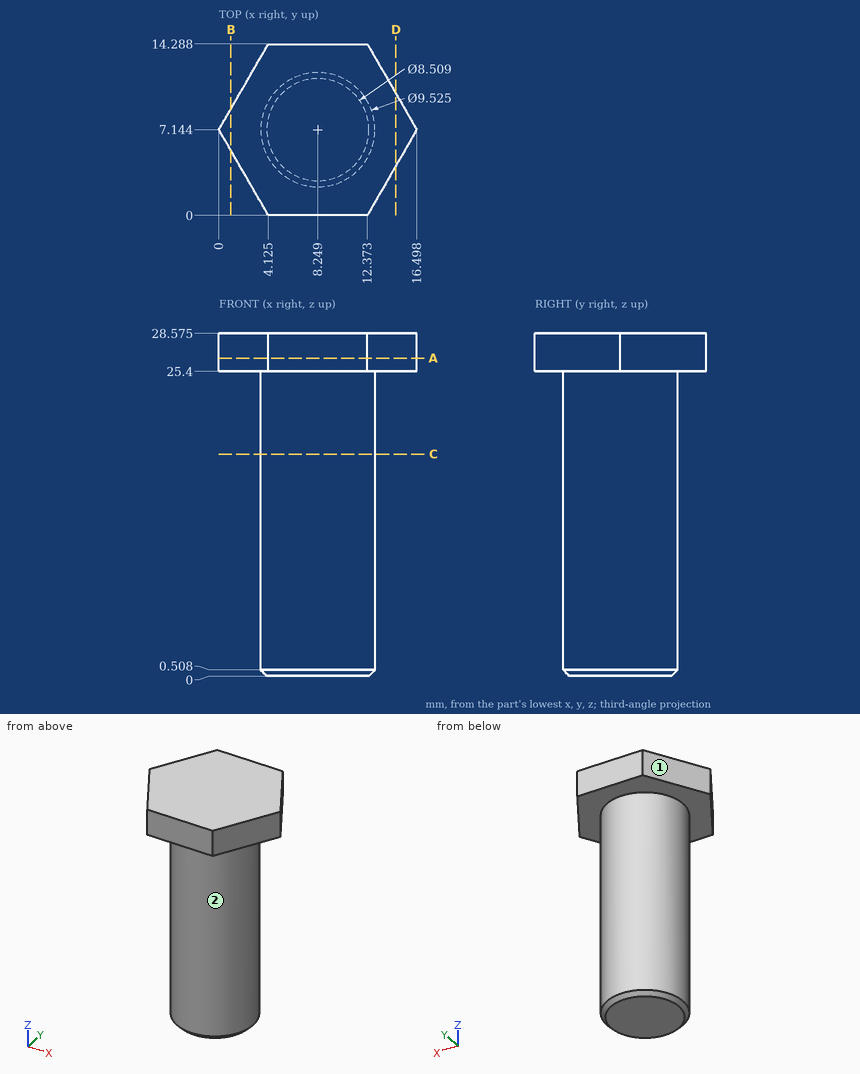
Part print with two shaded views. Sizes in mm from the minimum x, y, z corner. A direction names the side the tool comes from. Round coordinates to 2 decimals unless told otherwise and drop trailing zeros. Write each loop counter-clockwise with the first axis right and the second up, starting at its lowest first coordinate (ties: lowest second). Pieces come first, ordered by that corner, then holes. Notation, with made-up numbers: M 0,27.5 L 18,27.5 A26 cw 18,56.5 Z; hole C 74,35.5 d5. An arc over 180 degrees is marked long. Answer as CSV lines item,"result". Start each with the question number.
1) Which spindle directions (+Z, -Z, +X, -X, +Y, -Y) get a long thin tool onto all of the face, cutting with end or side? Do the marked faces 1 and 2. Say none if no direction does.
2) Band-saw the part on C-C (z = 18.5). List the corners of the cut face in (x, y) (1 decimal).
3) Drill centre lines: L1, parallel to Y at x = 13.75, z = 26.75 (1 decimal); L2, parallel to Z at x = 13, y = 11 (1 decimal); L3, parallel to X at y = 7, z = 20.5. Where is each one in solid material? Low to high.
4) Band-saw the part on B-B (x = 1). List the corners of the cut face in (y, z) (1 decimal), then the cut area to 3 significant figures.
5) Band-saw the part on A-A (z = 26.5). List the corners of the cut face in (x, y) (1 decimal).
6) Band-saw the part on D-D (x = 14.75). List the corners of the cut face in (y, z) (1 decimal), then the cut area to 3 significant figures.
7) Drop flat-ended pins along their axis: pin 1 (2 mm diameter, centred on y = 6.5, z = 11, fed in from +X); pin 2 (1.5 mm diameter, centred on y = 11, z = 22.5, fed in from -X); pin 3 (5 mm diameter, centred on y = 9, z = 21, fed in from -X). Give the stop position or say it passes through.
Worked out:
1,face 1,"+Z, -Z, -X, +Y"
1,face 2,"-Z"
2,outline,"C 8.2,7.1 d9.5"
3,L1,"2.4 to 11.9"
3,L2,"25.4 to 28.6"
3,L3,"3.49 to 13.01"
4,outline,"M 5.4,25.4 L 8.9,25.4 L 8.9,28.6 L 5.4,28.6 Z"
4,area,"11.0 mm²"
5,outline,"M 0,7.1 L 4.1,0 L 12.4,0 L 16.5,7.1 L 12.4,14.3 L 4.1,14.3 Z"
6,outline,"M 4.1,25.4 L 10.2,25.4 L 10.2,28.6 L 4.1,28.6 Z"
6,area,"19.2 mm²"
7,pin 1,"x = 13.01"
7,pin 2,"x = 4.64"
7,pin 3,"x = 3.49"
